```python
from build123d import *

# Parameters (mm, degrees)
SKETCH1_R           = 45
BOSS_EXTRUDE1_DEPTH = 40
FILLET1_R           = 5
SKETCH2_R           = 30
CUT_EXTRUDE1_DEPTH  = 15
FILLET2_R           = 2
SKETCH3_R           = 1.5
CUT_EXTRUDE2_DEPTH  = 2
SKETCH4_W           = 3
SKETCH4_H           = 3
BOSS_EXTRUDE2_DEPTH = 15


with BuildPart() as part:
    # Sketch1 → Boss-Extrude1 (new body)
    with BuildSketch(Plane(origin=(0, 0, 0), x_dir=(1, 0, 0), z_dir=(0, 1, 0))):
        Circle(SKETCH1_R)
    extrude(amount=BOSS_EXTRUDE1_DEPTH)

    # Fillet1
    fillet1_edges = [part.edges().sort_by_distance(p)[0] for p in [
        (-45, 0, 0),
        (-45, 40, 0),
    ]]
    fillet(fillet1_edges, radius=FILLET1_R)

    # Sketch2 → Cut-Extrude1 (cut)
    with BuildSketch(Plane(origin=(0, 40, 0), x_dir=(1, 0, 0), z_dir=(0, 1, 0))):
        Circle(SKETCH2_R)
    extrude(amount=-CUT_EXTRUDE1_DEPTH, mode=Mode.SUBTRACT)

    # Fillet2
    fillet2_edges = [part.edges().sort_by_distance(p)[0] for p in [
        (-30, 25, 0),
        (-30, 40, 0),
    ]]
    fillet(fillet2_edges, radius=FILLET2_R)

    # Sketch3 → Cut-Extrude2 (cut)
    with BuildSketch(Plane(origin=(0, 40, 0), x_dir=(1, 0, 0), z_dir=(0, 1, 0))):
        with Locations((0, 35.324029749)):
            Circle(SKETCH3_R)
        with Locations((20.762943738, 28.577740377)):
            Circle(SKETCH3_R)
        with Locations((33.595148675, 10.915725502)):
            Circle(SKETCH3_R)
        with Locations((33.595148675, -10.915725502)):
            Circle(SKETCH3_R)
        with Locations((20.762943738, -28.577740377)):
            Circle(SKETCH3_R)
        with Locations((0, -35.324029749)):
            Circle(SKETCH3_R)
        with Locations((-20.762943738, -28.577740377)):
            Circle(SKETCH3_R)
        with Locations((-33.595148675, -10.915725502)):
            Circle(SKETCH3_R)
        with Locations((-33.595148675, 10.915725502)):
            Circle(SKETCH3_R)
        with Locations((-20.762943738, 28.577740377)):
            Circle(SKETCH3_R)
    extrude(amount=-CUT_EXTRUDE2_DEPTH, mode=Mode.SUBTRACT)

    # Sketch4 → Boss-Extrude2 (add)
    with BuildSketch(Plane(origin=(0, 25, 0), x_dir=(1, 0, 0), z_dir=(0, 1, 0))):
        with Locations((0.059295031, 24)):
            Rectangle(SKETCH4_W, SKETCH4_H)
    extrude(amount=BOSS_EXTRUDE2_DEPTH)


solid = part.part
```
CAD build for the part. Positions are in the model's coordinates, mm. A direction names the side the tool comes from. Give positions to 0.01 mm unless a question says otherwise; leave off trailing zeros. Loops run counter-clockwise (first coordinate to the right, second up) from the corner with the lowest first, then second, coordinate; pieces in that order, holes last. Notation, with made-up numbers: (45.5, 5) -> (70.5, 5) arc R20 cw to (70.5, 42) -> close; hole circle Ø8 at (-28, -1). An arc over 180 degrees is marked (long way). Use a Markdown table: item, result.
1. Mould opens along Z. For faces 1 (the flat face through (-21, 38, 29)), 2 (the flat face through (18, 40, -27)) say: pulls with the +Z half, pulls with the -Z half, needs draft (parallel to the pull), parting line crosses it, or undercut.
Check result:
| item | result |
|---|---|
| face 1 | undercut |
| face 2 | needs draft |
2. Slice it at C-C (y = 13). List the corners of the cut face in (x, z).
Check result:
| item | result |
|---|---|
| outline | circle Ø90 at (0, 0) |
3. Slice it at B-B (z = 0). List the corners of the cut face in (x, y), plus the area to 3 significant figures.
Check result:
| item | result |
|---|---|
| outline | (-45, 5) arc R5 ccw to (-40, 0) -> (40, 0) arc R5 ccw to (45, 5) -> (45, 35) arc R5 ccw to (40, 40) -> (32, 40) arc R2 ccw to (30, 38) -> (30, 27) arc R2 cw to (28, 25) -> (-28, 25) arc R2 cw to (-30, 27) -> (-30, 38) arc R2 ccw to (-32, 40) -> (-40, 40) arc R5 ccw to (-45, 35) -> close |
| area | 2,680 mm^2 |
4. Which spindle directions (+Z, -Z, +X, -X, +Y, -Y) get a long thin tool onto all of the face, cutting with end or side? Do faces 3 (the cylindrical face through (-35.094, 39.014, -10.982)), 4 (the flat face through (-1, 0, -1)). Say none if no direction does.
Check result:
| item | result |
|---|---|
| face 3 | +Y |
| face 4 | +Z, -Z, +X, -X, -Y |
5. Flat gauge pins, fed straight in: pin 1 (6 mm diameter, centred on y = 18.5, z = -26.5, fed in from +X); pin 2 (1.5 mm diameter, centred on x = 21.5, z = -15.5, fed in from +Y); pin 3 (6 mm diameter, centred on x = -35.5, y = 24, fed in from -Z). Where does each tip first touch, or does it go through?
Check result:
| item | result |
|---|---|
| pin 1 | stops at x = 38.38 |
| pin 2 | stops at y = 25 |
| pin 3 | stops at z = -31.12 |
6. Slice it at A-A (x = 0). List the corners of the cut face in (y, z), plus the area to 3 significant figures.
Check result:
| item | result |
|---|---|
| outline | (0, -40) arc R5 ccw to (5, -45) -> (35, -45) arc R5 ccw to (40, -40) -> (40, -36.82) -> (38, -36.82) -> (38, -33.82) -> (40, -33.82) -> (40, -32) arc R2 ccw to (38, -30) -> (27, -30) arc R2 cw to (25, -28) -> (25, -25.5) -> (40, -25.5) -> (40, -22.5) -> (25, -22.5) -> (25, 28) arc R2 cw to (27, 30) -> (38, 30) arc R2 ccw to (40, 32) -> (40, 33.82) -> (38, 33.82) -> (38, 36.82) -> (40, 36.82) -> (40, 40) arc R5 ccw to (35, 45) -> (5, 45) arc R5 ccw to (0, 40) -> close |
| area | 2,710 mm^2 |
7. Wall check: L1, parallel to X at y = 33, z = 0; L2, parallel to Y at x = -5, z = 8; L3, parallel to X at y = 32, z = -22. Give the ranges that are in metal, low to high. Write a range as [from, to].
Check result:
| item | result |
|---|---|
| L1 | x = [-45, -30], [30, 45] |
| L2 | y = [0, 25] |
| L3 | x = [-39.26, -20.4], [20.4, 39.26] |
